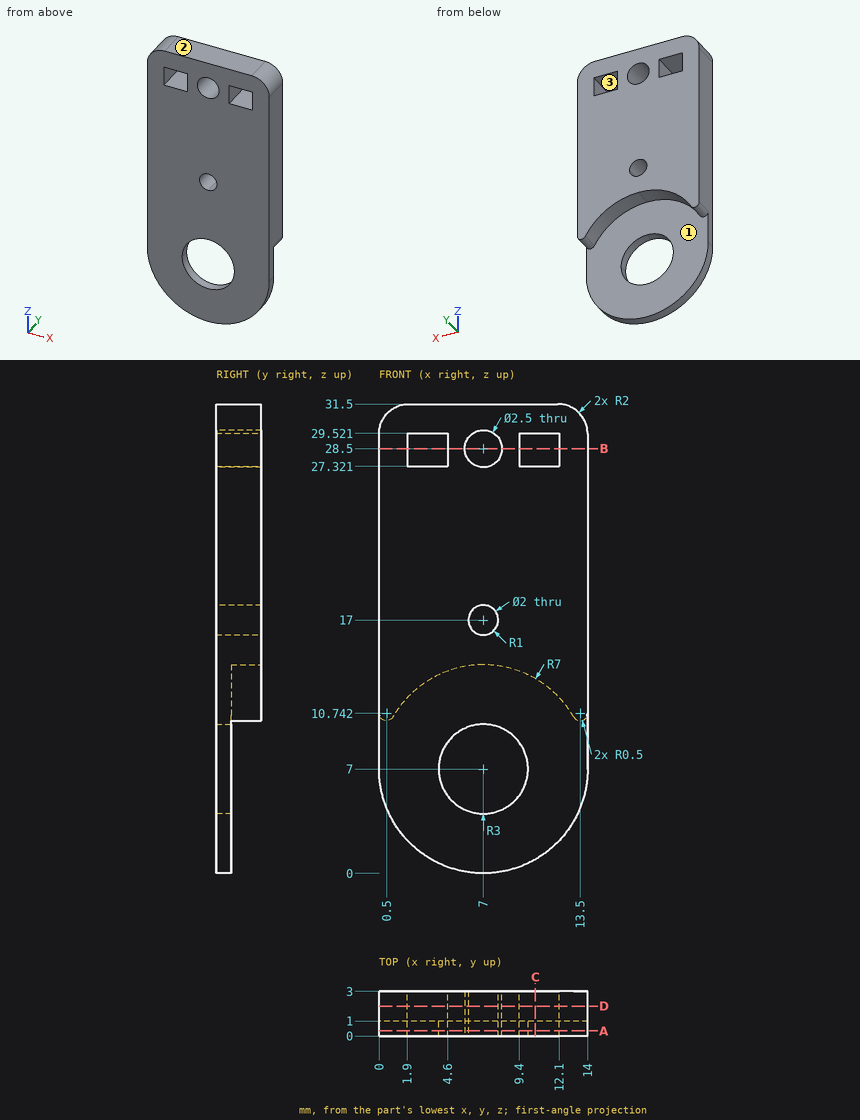
For this review, use the dimensioned drawing (mm, ordinates from the lowest corner) and the shaded views. A direction names the side the tool comes from. Round coordinates to 2 decimals unless told otherwise and drop trailing zeros. Write each loop counter-clockwise with the first axis right and the second up, starting at its lowest first coordinate (ties: lowest second). Pieces come first, ordered by that corner, then holes. Notation, with made-up numbers: M 31,5.25 L 39,5.25 A17 cw 39,26.25 Z; hole C 20.25,62 d9. An arc over 180 degrees is marked long. Write item = value, one per line. Start each with the question number.
(1) We need section D-D (y = 2). Give the boundary of the cut face in (x, z).
(2) For the marked faces 1, 2 and 3, list the 3-axis set-ups (+Z, -Z, +X, -X, +Y, -Y) from which the entire face can be reached by the end or side of a thin tool; tool diameter is ignored.
(3) We need section B-B (z = 28.5). Give the boundary of the cut face in (x, y), then the cut area to 3 significant figures.
(4) We need section A-A (y = 0.35). Give the boundary of the cut face in (x, z).
(5) For line 1 along Z through (x, y) = (7, 1.8); line 2 along X through (y, z) = (1.85, 28.5); line 3 along Z through (x, y) = (7, 0.7), list the stretches that pass through material, from the lowest coordinate up.
(6) We need section C-C (x = 10.5). Give the boundary of the cut face in (y, z).
(7) Clearance check with flat-ended pins moving along their axes: pin 1 Ø7 at (x, z) = (5.5, 8.5) entering from +Y; pin 2 Ø1.5 at (x, y) = (5, 0.5) entering from -Z. State where each tip first meets the part, or that it passes through.
Results found:
q1.outline = M 0,10.74 A0.5 ccw 0.93,10.49 A7 cw 13.07,10.49 A0.5 ccw 14,10.74 L 14,29.5 A2 ccw 12,31.5 L 2,31.5 A2 ccw 0,29.5 Z; hole M 1.9,27.32 L 4.6,27.32 L 4.6,29.52 L 1.9,29.52 Z; hole C 7,28.5 d2.5; hole C 7,17 d2; hole M 9.4,27.32 L 12.1,27.32 L 12.1,29.52 L 9.4,29.52 Z
q2.face_1 = -Z, +Y
q2.face_2 = +Z, +X, -X, +Y, -Y
q2.face_3 = +Y, -Y
q3.outline = M 0,0 L 1.9,0 L 1.9,3 L 0,3 Z; M 4.6,0 L 5.75,0 L 5.75,3 L 4.6,3 Z; M 8.25,0 L 9.4,0 L 9.4,3 L 8.25,3 Z; M 12.1,0 L 14,0 L 14,3 L 12.1,3 Z
q3.area = 18.3 mm²
q4.outline = M 0,7 A7 ccw 14,7 L 14,29.5 A2 ccw 12,31.5 L 2,31.5 A2 ccw 0,29.5 Z; hole M 1.9,27.32 L 4.6,27.32 L 4.6,29.52 L 1.9,29.52 Z; hole C 7,7 d6; hole C 7,28.5 d2.5; hole C 7,17 d2; hole M 9.4,27.32 L 12.1,27.32 L 12.1,29.52 L 9.4,29.52 Z
q5.line_1 = 14 to 16, 18 to 27.25, 29.75 to 31.5
q5.line_2 = 0 to 1.9, 4.6 to 5.75, 8.25 to 9.4, 12.1 to 14
q5.line_3 = 0 to 4, 10 to 16, 18 to 27.25, 29.75 to 31.5
q6.outline = M 0,0.94 L 1,0.94 L 1,13.06 L 3,13.06 L 3,27.32 L 0,27.32 Z; M 0,29.52 L 3,29.52 L 3,31.5 L 0,31.5 Z
q7.pin_1 = 1
q7.pin_2 = 0.11
